Verification items for the finished model (mm, model axes). Face numbers are marked on the shaded views. A direction names the side the tool comes from. Give positions to 0.01 mm unless a question says otherwise; leave off trailing zeros. Write each loop counter-clockwise with the first axis right and the second up, starting at its lowest first coordinate (ties: lowest second). Pieces come first, ordered by that corner, then holes. Notation, with made-up numbers: (67.5, -19) -> (96.5, -19) arc R11 cw to (96.5, -5) -> close; hole circle Ø10 at (35.5, 34). An arc over 180 degrees is marked (long way). Write item = value, one per line.
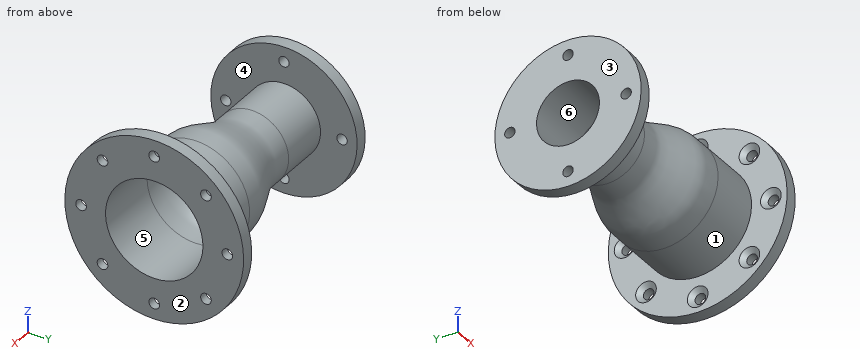
from build123d import *

# Parameters (mm, degrees)
CSK_FOR_5_8_FLAT_HEAD_MACHINE_SCREW_100_D           = 16.66748
CSK_FOR_5_8_FLAT_HEAD_MACHINE_SCREW_100_DEPTH       = 20
CSK_FOR_5_8_FLAT_HEAD_MACHINE_SCREW_100_CSINK_D     = 32.3088
CSK_FOR_5_8_FLAT_HEAD_MACHINE_SCREW_100_CSINK_ANGLE = 100
F_5_8_CLEARANCE_HOLE1_D                             = 16.27124
F_5_8_CLEARANCE_HOLE1_DEPTH                         = 20


with BuildPart() as part:
    # Sketch2 → Revolve1 (revolve)
    with BuildSketch(Plane.XY, mode=Mode.PRIVATE) as revolve1_sk:
        with BuildLine():
            Line((341.7, 76.137499212), (341.7, 139.7))
            Line((341.7, 139.7), (321.7, 139.7))
            Line((321.7, 139.7), (321.7, 84.137499212))
            Line((321.7, 84.137499212), (238.7, 84.137499212))
            add(Edge.make_bspline(
                [(238.7, 84.137499212), (238.355924075, 84.137499212), (237.667772223, 84.137499211), (236.43892963, 84.137499212), (234.866011112, 84.137499209), (233.096477778, 84.137499221), (231.179483334, 84.137499181), (229.409949997, 84.137499346), (227.492955565, 84.137498785), (225.723422181, 84.137501116), (223.806427909, 84.137493202), (222.03689386, 84.137526067), (220.119901847, 84.137414453), (218.350358415, 84.137877999), (216.436180482, 84.136306025), (214.671251811, 84.142808495), (212.761120781, 84.086749305), (210.997970421, 83.981894478), (209.088061418, 83.811610968), (207.325068085, 83.603702947), (205.415339805, 83.325577691), (203.652528826, 83.021476856), (201.742980231, 82.643054651), (199.980349522, 82.250081454), (198.070973132, 81.779589057), (196.308510241, 81.305636666), (194.399291637, 80.751921317), (192.636978054, 80.205434277), (190.727898375, 79.577923288), (188.965712472, 78.967858654), (187.056750607, 78.276511422), (185.294669761, 77.61229035), (183.385803915, 76.867540678), (181.623805854, 76.15899109), (179.715014471, 75.371680114), (177.95307795, 74.628970979), (176.044340155, 73.810271455), (174.28244512, 73.043839656), (172.373740784, 72.205172954), (170.611868192, 71.425644088), (168.701772289, 70.577967809), (166.937395899, 69.794959659), (165.024786727, 68.949453647), (163.259291454, 68.174390413), (161.346657228, 67.343861664), (159.58112861, 66.587981326), (157.668449277, 65.784003027), (155.902867536, 65.057899506), (153.990122343, 64.291832507), (152.22446654, 63.60586364), (150.311633974, 62.888769921), (148.545882008, 62.252980739), (146.632940071, 61.595543531), (144.867069113, 61.019596499), (142.95399603, 60.432048638), (141.187983586, 59.925161995), (139.274759098, 59.417223546), (137.508584813, 58.988118492), (135.595192141, 58.568944237), (133.828840435, 58.225800875), (131.915268777, 57.903938632), (130.148732425, 57.654357312), (128.234978669, 57.437727635), (126.468267149, 57.288649922), (124.789582716, 57.197477456), (123.443760708, 57.156958736), (122.420535806, 57.149027418), (121.677966993, 57.150148752), (120.601758891, 57.149831794), (119.202172332, 57.150049881), (117.285177742, 57.149983489), (115.515644452, 57.150003038), (113.598649997, 57.149998331), (111.829116667, 57.149999717), (109.912122221, 57.149999383), (108.142588888, 57.149999482), (106.225594444, 57.149999458), (104.45606111, 57.149999465), (102.539066666, 57.149999463), (101.039878703, 57.149999464), (99.81103611, 57.149999464), (99.27034537, 57.149999464), (98.999999999, 57.149999464)],
                knots=[0, 0, 0, 0, 0.007154165, 0.014308329, 0.025550588, 0.039858917, 0.051101176, 0.065409505, 0.076651764, 0.090960094, 0.102202352, 0.116510682, 0.12775294, 0.14206127, 0.153303528, 0.167554008, 0.178755429, 0.193030915, 0.204271905, 0.218620642, 0.229935227, 0.24439542, 0.255809505, 0.270408809, 0.281939941, 0.296695409, 0.308352907, 0.323271342, 0.335056718, 0.350135378, 0.362042998, 0.377270556, 0.389288475, 0.404646168, 0.416757099, 0.432220021, 0.44440238, 0.459940864, 0.472169892, 0.487750951, 0.499999862, 0.51562065, 0.52788688, 0.543480107, 0.55571106, 0.571242545, 0.583412274, 0.598850533, 0.610935794, 0.626253518, 0.638234915, 0.653410393, 0.66527347, 0.680291945, 0.692028204, 0.706883096, 0.718490902, 0.733184872, 0.744670204, 0.75921598, 0.770592966, 0.785013865, 0.796305044, 0.810635098, 0.821871343, 0.831256632, 0.838627865, 0.843146285, 0.846696472, 0.861004801, 0.87224706, 0.886555389, 0.897797648, 0.912105977, 0.923348236, 0.937656565, 0.948898824, 0.963207153, 0.974449412, 0.988757741, 0.994378871, 1, 1, 1, 1], degree=3, weights=[0.576132148, 0.576132148, 0.576132148, 0.576132148, 0.576132148, 0.576132148, 0.576132148, 0.576132148, 0.576132148, 0.576132148, 0.576132148, 0.576132148, 0.576132148, 0.576132148, 0.576132148, 0.576132148, 0.576132148, 0.576132148, 0.576132148, 0.576132148, 0.576132148, 0.576132148, 0.576132148, 0.576132148, 0.576132148, 0.576132148, 0.576132148, 0.576132148, 0.576132148, 0.576132148, 0.576132148, 0.576132148, 0.576132148, 0.576132148, 0.576132148, 0.576132148, 0.576132148, 0.576132148, 0.576132148, 0.576132148, 0.576132148, 0.576132148, 0.576132148, 0.576132148, 0.576132148, 0.576132148, 0.576132148, 0.576132148, 0.576132148, 0.576132148, 0.576132148, 0.576132148, 0.576132148, 0.576132148, 0.576132148, 0.576132148, 0.576132148, 0.576132148, 0.576132148, 0.576132148, 0.576132148, 0.576132148, 0.576132148, 0.576132148, 0.576132148, 0.576132148, 0.576132148, 0.576132148, 0.576132148, 0.576132148, 0.576132148, 0.576132148, 0.576132148, 0.576132148, 0.576132148, 0.576132148, 0.576132148, 0.576132148, 0.576132148, 0.576132148, 0.576132148, 0.576132148, 0.576132148]))
            Line((98.999999999, 57.149999464), (20, 57.149999464))
            Line((20, 57.149999464), (20, 114.3))
            Line((20, 114.3), (0, 114.3))
            Line((0, 114.3), (0, 49.149999464))
            Line((0, 49.149999464), (98.999999999, 49.149999464))
            add(Edge.make_bspline(
                [(238.700000001, 76.137499212), (235.69409428, 76.137499211), (231.185175342, 76.137529978), (225.92498116, 76.137458281), (222.918904328, 76.137568327), (220.664664612, 76.137283149), (218.784669959, 76.138023248), (217.290602157, 76.13677783), (216.128457097, 76.1382361), (215.066881493, 76.138852647), (213.792519107, 76.118938664), (211.496695076, 76.015652057), (208.229301379, 75.6893674), (204.270612611, 75.027164667), (200.298712296, 74.120693109), (194.985358164, 72.623109637), (188.321466773, 70.283294689), (180.275439823, 66.96143105), (172.126179657, 63.34551056), (163.790302615, 59.64532736), (155.164556548, 56.079333574), (147.64132386, 53.429737774), (141.378908996, 51.662061148), (136.556364248, 50.559794229), (131.615917341, 49.730227773), (127.403841781, 49.309288048), (124.437765649, 49.174559905), (122.930150126, 49.151400947), (122.100741829, 49.149426118), (121.356980871, 49.150399773), (120.417271001, 49.149754665), (118.913072261, 49.150117503), (117.035873074, 49.149952223), (114.780889972, 49.150013449), (111.775161973, 49.149990987), (106.514717734, 49.150005821), (102.005905795, 49.149999464), (98.999999999, 49.149999464)],
                knots=[0, 0, 0, 0, 0.0625, 0.09375, 0.109375, 0.125, 0.140625, 0.1484375, 0.15625, 0.1640625, 0.171875, 0.1875, 0.21875, 0.25, 0.28125, 0.3125, 0.375, 0.4375, 0.5, 0.5625, 0.625, 0.6875, 0.71875, 0.75, 0.78125, 0.8125, 0.828125, 0.8359375, 0.83984375, 0.84375, 0.8515625, 0.859375, 0.875, 0.890625, 0.90625, 0.9375, 1, 1, 1, 1], degree=3))
            Line((238.700000001, 76.137499212), (341.7, 76.137499212))
        make_face()
    revolve(revolve1_sk.sketch.rotate(Axis((341.7, 0, 0), (-1, 0, 0)), 90), axis=Axis((341.7, 0, 0), (-1, 0, 0)))

    # CSK for 5_8 Flat Head Machine Screw _100
    with Locations(Plane(origin=(321.7, -86.94526051, 61.229912904), x_dir=(0, 0, 1), z_dir=(-1, 0, 0))):
        with Locations((-61.229912904, 201.24526051), (-176.596487394, 86.94526051), (-142.052217993, 167.767565599), (19.592392186, 167.767565599), (53.070087096, 86.94526051), (19.592392186, 6.12295542), (-61.229912904, -27.406492985), (-142.052217993, 6.12295542)):
            CounterSinkHole(CSK_FOR_5_8_FLAT_HEAD_MACHINE_SCREW_100_D / 2, CSK_FOR_5_8_FLAT_HEAD_MACHINE_SCREW_100_CSINK_D / 2, depth=CSK_FOR_5_8_FLAT_HEAD_MACHINE_SCREW_100_DEPTH, counter_sink_angle=CSK_FOR_5_8_FLAT_HEAD_MACHINE_SCREW_100_CSINK_ANGLE)

    # 5/8 Clearance Hole1
    with Locations(Plane(origin=(0, -86.94526051, 61.229912904), x_dir=(0, 0, 1), z_dir=(-1, 0, 0))):
        with Locations((-61.229912904, 177.798020209), (29.681467244, 86.94526051), (-61.229912904, -3.966119638), (-152.141293051, 86.94526051)):
            Hole(F_5_8_CLEARANCE_HOLE1_D / 2, depth=F_5_8_CLEARANCE_HOLE1_DEPTH)


solid = part.part
Item 1: Sectioned sample at B-B on z = 0. Give the number of separate pieces and of enclosed holes in the cut face, then the cut area to 3 significant figures.
Response values:
separate_pieces = 6
enclosed_holes = 0
area = 8,630 mm^2
Item 2: Material ranges on line 1 (Y direction, x = 7, z = 0); line 2 (X direction, y = 93, z = 23); line 3 (Y direction, x = 337, z = 0), recorded low to high.
Response values:
line_1 = -114.3 to -99.05, -82.78 to -49.15, 49.15 to 82.72, 98.99 to 114.3
line_2 = 0 to 20, 321.7 to 341.7
line_3 = -139.7 to -122.69, -106.02 to -76.14, 76.14 to 105.97, 122.63 to 139.7
Item 3: Sectioned sample at D-D on x = 34.5. Record the cut outline in (y, z).
Response values:
outline = circle Ø114.3 at (0, 0); hole circle Ø98.3 at (0, 0)
Item 4: Sectioned sample at A-A on x = 248. Record the cut outline in (y, z) (1 decimal), then the cut area to 3 significant figures.
Response values:
outline = circle Ø168.3 at (0, 0); hole circle Ø152.3 at (0, 0)
area = 4,030 mm^2
Item 5: Mould release check, pull along X, two halves, no side actions. Record for the marked faces 1, 2 and 3: +X half, -X half, draft (parallel to the pull), parting line (faces both ways), or undercut.
Response values:
face_1 = undercut
face_2 = +X half
face_3 = -X half
Item 6: Go/stop test with flat-tipped pins: P1, Ø13.5, axis at y = 80.82, z = -80.82, coming from the +X side; P2, Ø12, axis at x = 223, z = -71.5, coming from the -Y side; P3, Ø13, axis at y = -90.91, z = 0, coming from the -X side. Record where each tip stops, or that it passes through.
Response values:
P1 = 20
P2 = -52.81
P3 = 321.7
Item 7: Set-up check for the marked faces 4, 5 and 6: record each of +Z, -Z, +X, -X, +Y, -Y from which the full face is reachable in a straight line by a thin tool's end or side.
Response values:
face_4 = none
face_5 = +X
face_6 = +X, -X
